Check sheet for the modelled part. Datum: model origin and axes. Units: mm. A direction names the side the tool comes from. Round coordinates to 2 decimals unless told otherwise and drop trailing zeros. Order: outer loops, then holes, each group sorted by start corner. A loop starts at its lowest first (then second) coordinate and runs counter-clockwise, first axis right, second up. Notation, with made-up numbers: (35.25, 8.5) -> (74.25, 8.5) arc R19 cw to (74.25, 37.5) -> close; hole circle Ø4 at (-24.75, 17.25). An arc over 180 degrees is marked (long way). Use CSV: the item, a comma, the result in double quotes.
Autodesk Fusion 360 part; units mm, degrees
sketch "Sketch1" plane through (0, 0, 0) normal (0, 0, 1) x (1, 0, 0)
  circle A0 centre (0, 0) radius 5.3
  circle A1 centre (0, 0) radius 8.05
  circle A2 centre (0, 0) radius 10.35
  circle A3 centre (0, 0) radius 2.5
  circle A4 centre (0, 0) radius 3
  dimension "d1" = 10.6
  dimension "d2" = 16.1
  dimension "d3" = 20.7
  dimension "d8" = 5
  dimension "d9" = 6
extrude "Extrude1" add sketch "Sketch1" along normal blind 30 contours A0 | A2 | A4 makes body 1 at (10.2986, -1.0305, 20) makes body 2 at (5.2737, -0.5277, 20)
extrude "Extrude2" add sketch "Sketch1" along normal blind 28 contours A1 bodies 1 2
extrude "Extrude3" cut sketch "Sketch1" along normal blind 25 contours A3 | A4 bodies 1
chamfer "Chamfer1" distance 1 distance2 10 1 edges at (-9.6496, -3.7427, 30) measured on face at (9.5148, -0.9141, 30) on bodies 1
sketch "Sketch2" plane through (0, 0, 0) normal (1, 0, 0) x (0, 0, -1)
  arc A0 (-38, -10) -> (-28, 0) centre (-38, 0) ccw
  line L0 (-28, 0) -> (-38, 0)
  line L1 (-38, 0) -> (-38, -10)
  line L2 (-1.75, 0) -> (-22.5, 0)
  dimension "d14" = 10
  dimension "d15" = 38
revolve "Revolve1" cut sketch "Sketch2" angle 360 about axis through (0, 0, 28) along (0, 0, 1) bodies 1
equation "d8 = draadstang - 2 * draadstangtolerance"
equation "d9 = draadstang"
equation "draadstang = 6 mm"
equation "draadstangtolerance = 0.5 mm"
Q1. Scan lines: L1, parallel to Y at x = 0, z = 15; L2, parallel to Y at x = 0, z = 29.4; L3, parallel to Y at x = 0, z = 28.8. Record each from-to range of solid material in increasing order.
Result sheet:
L1,"y = -10.35 to -3, 3 to 10.35"
L2,"y = -9.41 to -8.05, -5.3 to -5.1, 5.1 to 5.3, 8.05 to 9.41"
L3,"y = -9.47 to -8.05, -5.3 to -3.92, 3.92 to 5.3, 8.05 to 9.47"
Q2. Sectioned sample at C-C, the plane z = 9.25. Enter the section's corners in (x, y), then the cut area to 3 significant figures.
Result sheet:
outline,"circle Ø20.7 at (0, 0); hole circle Ø6 at (0, 0)"
area,"308 mm^2"
Q3. Go/stop test with flat-tipped pins: pin 1 (8 mm diameter, centred on x = 0, y = 0, fed in from -Z); pin 2 (3 mm diameter, centred on y = 5, z = 11, fed in from +X); pin 3 (1.5 mm diameter, centred on y = 6.5, z = 24.5, fed in from -X); pin 4 (2 mm diameter, centred on y = 1.5, z = 24.5, fed in from -X). Record where each tip stops, or that it passes through.
Result sheet:
pin 1,"stops at z = 0"
pin 2,"stops at x = 9.74"
pin 3,"stops at x = -8.07"
pin 4,"stops at x = -9.94"
Q4. Mould release check, pull along Y, two halves, no side actions. Record for faces 4 (the face through (3, 8, 30)), 5 (the face through (9.296, -2.927, 26.041)), 6 (the face through (7.678, -2.418, 28.986)): pulls with the +Y half, pulls with the -Y half, needs draft (parallel to the pull), parting line crosses it, or undercut.
Result sheet:
face 4,"needs draft"
face 5,"parting line crosses it"
face 6,"undercut"
Q5. Sectioned sample at A-A, the plane y = 0. Enter the section's corners in (x, z), then the cut area to 3 significant figures.
Result sheet:
outline,"(-10.35, 0) -> (-3, 0) -> (-3, 25) -> (-2.5, 25) -> (-2.5, 28.32) arc R10 cw to (-5.3, 29.52) -> (-5.3, 28) -> (-8.05, 28) -> (-8.05, 30) -> (-9.35, 30) -> (-10.35, 20) -> close; (2.5, 25) -> (3, 25) -> (3, 0) -> (10.35, 0) -> (10.35, 20) -> (9.35, 30) -> (8.05, 30) -> (8.05, 28) -> (5.3, 28) -> (5.3, 29.52) arc R10 cw to (2.5, 28.32) -> close"
area,"418 mm^2"
Q6. Access from +Z, -Z, +X, -X, +Y, -Y to the whole of each face (thin tool, end or side, straight path). Record for faces 1 (the face through (-2.4, -2.2, 0)), 2 (the face through (4.896, 2.03, 28.749)), 3 (the face through (-3, 0, 12)).
Result sheet:
face 1,"-Z, +X, -X, +Y, -Y"
face 2,"+Z"
face 3,"-Z"
